```python
from build123d import *

# Parameters (mm, degrees)
F1_DEPTH = 15
F2_R     = 0.99999


# Not quite as in the source:
# - a fillet or chamfer is up to 0.001 mm smaller than in the source, because OpenCascade refuses the exact size


with BuildPart() as f1:
    # F0 (on Top) → F1 (new body)
    with BuildSketch(Plane.XY):
        with BuildLine():
            ThreePointArc((-4.8464827516, -10.9777777778), (-2.4720661624, -10.2468824829), (0, -10))
            ThreePointArc((0, -10), (2.4720661624, -10.2468824829), (4.8464827516, -10.9777777778))
            ThreePointArc((4.8464827516, -10.9777777778), (10.0538001029, -6.5514199598), (12, 0))
            ThreePointArc((12, 0), (-6.5514199598, 10.0538001029), (-4.8464827516, -10.9777777778))
        make_face()
        with BuildLine():
            ThreePointArc((0, -10), (-7.0710678119, 7.0710678119), (10, 0))
            ThreePointArc((10, 0), (7.0710678119, -7.0710678119), (0, -10))
        make_face(mode=Mode.SUBTRACT)
        with BuildLine():
            ThreePointArc((4.8464827516, -10.9777777778), (2.4720661624, -10.2468824829), (0, -10))
            ThreePointArc((0, -10), (-2.4720661624, -10.2468824829), (-4.8464827516, -10.9777777778))
            ThreePointArc((-4.8464827516, -10.9777777778), (-2.4765567495, -11.7416637095), (0, -12))
            ThreePointArc((0, -12), (2.4765567495, -11.7416637095), (4.8464827516, -10.9777777778))
        make_face()
        with BuildLine():
            ThreePointArc((12.5, -22.5), (10.412277234, -15.5837522599), (4.8464827516, -10.9777777778))
            ThreePointArc((4.8464827516, -10.9777777778), (2.4765567495, -11.7416637095), (0, -12))
            ThreePointArc((0, -12), (7.4246212025, -15.0753787975), (10.5, -22.5))
            ThreePointArc((10.5, -22.5), (10.0140279829, -25.6574108948), (8.601096465, -28.5225525817))
            Line((8.601096465, -28.5225525817), (10.2394005536, -29.6697054544))
            ThreePointArc((10.2394005536, -29.6697054544), (11.9214618844, -26.2588224938), (12.5, -22.5))
        make_face()
        with BuildLine():
            ThreePointArc((0, -12), (-2.4765567495, -11.7416637095), (-4.8464827516, -10.9777777778))
            ThreePointArc((-4.8464827516, -10.9777777778), (-12.0101211002, -19.034889445), (-10.2394005536, -29.6697054544))
            Line((-10.2394005536, -29.6697054544), (-8.601096465, -28.5225525817))
            ThreePointArc((-8.601096465, -28.5225525817), (-9.3136137484, -17.651639561), (0, -12))
        make_face()
    extrude(amount=F1_DEPTH)

    # F2 (radius 1 in the source; OpenCascade refuses exactly that, so slightly less here)
    f2_edges = [f1.edges().sort_by_distance(p)[0] for p in [
        (-8.601096, -28.522553, 7.5),
        (-10.239401, -29.669705, 7.5),
        (8.601096, -28.522553, 7.5),
        (10.239401, -29.669705, 7.5),
    ]]
    fillet(f2_edges, radius=F2_R)


solid = f1.part
```
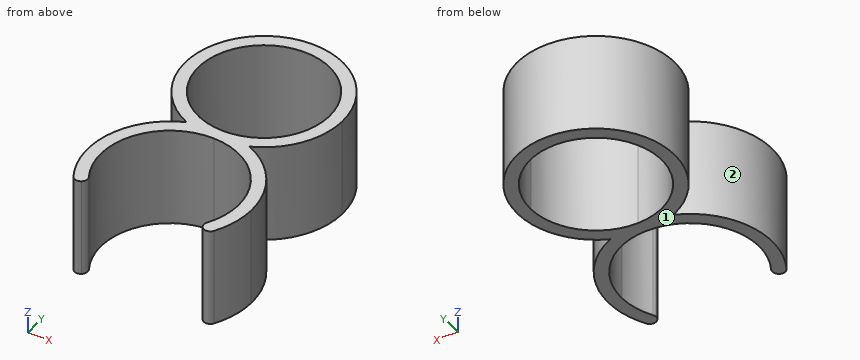
Could you check a few things on this model? Use its own coordinates, in mm. Face numbers are marked on the shaded views. Give positions to 0.01 mm unless a question says otherwise; leave off trailing zeros. Write each loop counter-clockwise with the first axis right and the second up, starting at its lowest first coordinate (ties: lowest second). Pieces come first, ordered by that corner, then holes. Notation, with made-up numbers: (-6.5, 89.5) - (36.5, 89.5) arc R24 ccw to (36.5, 109.5) - close; hole circle Ø5 at (64.25, 19.25). An arc over 180 degrees is marked (long way). One line per item, written item: value. Start each with the question number.
Item 1: Imagine slicing it at A-A, the plane x = -1.5. List the corners of the cut face in (y, z) for me, and give its area (3 significant figures).
Item 2: Please list where these lines run through material, in increasing order: line 1 (Y direction, x = 0, z = 10); line 2 (Y direction, x = -5.25, z = 4); line 3 (Y direction, x = 11, z = 12.5). Write a range as from..to.
Item 3: Imagine slicing it at C-C, the plane x = -7.75. List the corners of the cut face in (y, z) for me, and give its area (3 significant figures).
Item 4: I'm going to push flat-ended pins straight in: pin 1 (2 mm diameter, centred on y = -5, z = 10.5, fed in from -X); pin 2 (4 mm diameter, centred on x = 1.5, y = -6, fed in from +Z); pin 3 (1.5 mm diameter, centred on x = -7.5, z = 7, fed in from +Y); pin 4 (3 mm diameter, centred on y = -19, z = 12, fed in from +X). Where does each tip first touch, or does it pass through?
Item 5: Imagine slicing it at B-B, the plane y = -24. List the corners of the cut face in (x, z) for me, and give its area (3 significant figures).
Item 6: If we mould it in two halves opening along Y, with no side actions, what happens to the marked faces 1 and 2? For each: +Y half, -Y half, draft (parallel to the pull), parting line (faces both ways), or undercut.
Geometry says:
1. outline: (-12.11, 0) - (-9.89, 0) - (-9.89, 15) - (-12.11, 15) - close; (9.89, 0) - (11.91, 0) - (11.91, 15) - (9.89, 15) - close
1. area: 63.6 mm^2
2. line 1: -12..-10, 10..12
2. line 2: -13.41..-11.16, -10.79..-8.51, 8.51..10.79
2. line 3: -28.44..-16.56, -4.8..4.8
3. outline: (-15.42, 0) - (-12.69, 0) - (-12.69, 15) - (-15.42, 15) - close; (-9.16, 0) - (-6.32, 0) - (-6.32, 15) - (-9.16, 15) - close; (6.32, 0) - (9.16, 0) - (9.16, 15) - (6.32, 15) - close
3. area: 126 mm^2
4. pin 1: x = -11.31
4. pin 2: through
4. pin 3: y = 9.92
4. pin 4: x = 12.34
5. outline: (-12.41, 0) - (-10.39, 0) - (-10.39, 15) - (-12.41, 15) - close; (10.39, 0) - (12.41, 0) - (12.41, 15) - (10.39, 15) - close
5. area: 60.5 mm^2
6. face 1: draft
6. face 2: undercut
